Read the model definition and answer for the solid it produces. Units are mm, in the model's axes. A direction names the side the tool comes from. Give positions to 0.01 mm unless a question says otherwise; leave off trailing zeros. Write each loop counter-clockwise with the first axis right and the second up, starting at its lowest first coordinate (ties: lowest second). Pieces come first, ordered by that corner, then holes. Notation, with made-up numbers: (62, -18.5) - (115, -18.5) arc R20 cw to (115, 1.5) - close; hole circle Ø9 at (31.5, 79). An arc over 180 degrees is marked (long way). Answer as CSV lines item,"result".
Autodesk Inventor part; units mm, degrees
ref_plane "YZ Plane" through (0, 0, 0) normal (1, 0, 0) x (0, 1, 0)
ref_plane "XZ Plane" through (0, 0, 0) normal (0, 1, 0) x (-1, 0, 0)
ref_plane "XY Plane" through (0, 0, 0) normal (0, 0, 1) x (1, 0, 0)
sketch "Эскиз1" plane through (0, 0, 0) normal (0, 1, 0) x (-1, 0, 0)
  line L0 (0, 0) -> (90, 0)
  line L1 (90, 0) -> (90, -20)
  line L2 (90, -20) -> (6, -20)
  line L3 (0, 0) -> (0, -120)
  line L4 (0, -120) -> (90, -120)
  line L5 (90, -120) -> (90, -100)
  line L6 (90, -100) -> (6, -100)
  line L7 (6, -100) -> (6, -20)
  line L8 (90, 0) -> (90, -10)
  line L9 (90, -10) -> (80, -10)
  line L10 (90, -100) -> (90, -110)
  line L11 (90, -110) -> (80, -110)
  circle A0 centre (80, -10) radius 5
  circle A1 centre (80, -110) radius 5
  dimension "d4" = 90
  dimension "d5" = 20
  dimension "d6" = 84
  dimension "d7" = 120
  dimension "d8" = 20
  dimension "d9" = 10
  dimension "d10" = 10
  dimension "d11" = 10
  dimension "d12" = 10
  dimension "d13" = 10
  dimension "d14" = 10
extrude "Выдавливание1" add sketch "Эскиз1" along normal blind 20
sketch "Эскиз2" plane through (-6, 0, -100) normal (-1, 0, 0) x (0, 0, 1)
  line L0 (80, 0) -> (80, 20)
  line L1 (80, 0) -> (80, 10)
  line L2 (80, 10) -> (0, 10)
  line L3 (0, 0) -> (0, 20)
  circle A0 centre (40, 10) radius 3.5
  line L4 (40, 10) -> (60, 10)
  circle A1 centre (60, 10) radius 3.5
  line L5 (40, 10) -> (20, 10)
  circle A2 centre (20, 10) radius 3.5
  point P0 (100, 0)
  dimension "d17" = 7
  dimension "d18" = 20
  dimension "d19" = 7
  dimension "d20" = 20
  dimension "d21" = 7
extrude "Выдавливание2" cut sketch "Эскиз2" against normal blind 95.75
properties part number "Скоба для полки"
(1) Find the intervals of material crossed by L1, parallel to Z at x = -80, y = 15; L2, parallel to Z at x = -3.1, y = 10; L3, parallel to Y at x = -3.8, z = -60, in increasing order.
Worked out:
L1,"z = -120 to -115, -105 to -100, -20 to -15, -5 to 0"
L2,"z = -120 to -83.5, -76.5 to -63.5, -56.5 to -43.5, -36.5 to 0"
L3,"y = 0 to 6.5, 13.5 to 20"
(2) For faces 1 (the cylindrical face through (-84.619, 9.86, -108.085)), 2 (the flat face through (-49, 10, -100)), determine the directions among +Z, -Z, +X, -X, +Y, -Y from which every point of the face is accessible in a straight line to the end or side of a thin tool.
Worked out:
face 1,"+Y, -Y"
face 2,"-X, +Y, -Y"
(3) A cutting plane is placed at A-A (y = 10). Write down the section's boundary in (x, z).
Worked out:
outline,"(-90, -120) - (0, -120) - (0, -83.5) - (-6, -83.5) - (-6, -100) - (-90, -100) - close; (-90, -20) - (-6, -20) - (-6, -36.5) - (0, -36.5) - (0, 0) - (-90, 0) - close; (-6, -76.5) - (0, -76.5) - (0, -63.5) - (-6, -63.5) - close; (-6, -56.5) - (0, -56.5) - (0, -43.5) - (-6, -43.5) - close; hole circle Ø10 at (-80, -110); hole circle Ø10 at (-80, -10)"
(4) A cutting plane is placed at B-B (z = -60). Write down the section's boundary in (x, y), and give its area (3 significant figures).
Worked out:
outline,"(-6, 0) - (0, 0) - (0, 6.5) - (-6, 6.5) - close; (-6, 13.5) - (0, 13.5) - (0, 20) - (-6, 20) - close"
area,"78.0 mm^2"
(5) A cutting plane is placed at C-C (x = -80). Write down the section's boundary in (y, z), and give its area (3 significant figures).
Worked out:
outline,"(0, -120) - (20, -120) - (20, -115) - (0, -115) - close; (0, -105) - (20, -105) - (20, -100) - (0, -100) - close; (0, -20) - (20, -20) - (20, -15) - (0, -15) - close; (0, -5) - (20, -5) - (20, 0) - (0, 0) - close"
area,"400 mm^2"
(6) A cutting plane is placed at D-D (x = -9.5). Write down the section's boundary in (y, z), and give its area (3 significant figures).
Worked out:
outline,"(0, -120) - (20, -120) - (20, -100) - (0, -100) - close; (0, -20) - (20, -20) - (20, 0) - (0, 0) - close"
area,"800 mm^2"
(7) The mould has two halves that part along Z. Classify faces 3 (the flat face through (-44, 10, 0)), 4 (the flat face through (-44, 10, -120)), 5 (the cylindrical face through (-3, 7.9, -42.8)), 6 (the flat face through (-34, 0, -19)): +Z half, -Z half, draft (parallel to the pull), parting line (faces both ways), or undercut.
Worked out:
face 3,"+Z half"
face 4,"-Z half"
face 5,"undercut"
face 6,"draft"
(8) Each of these flat-tipped pins is pushed along its axis until it touches: P1, Ø16, axis at x = -80, z = -110, coming from the +Y side; P2, Ø11, axis at y = 10, z = -40, coming from the -X side; P3, Ø8, axis at x = -80, z = -10, coming from the -Y side. Where does it stop, or does it pass through?
Worked out:
P1,"stops at y = 20"
P2,"stops at x = -6"
P3,"passes through"
